from build123d import *

# Parameters (mm, degrees)
F1_DEPTH = 25.4


with BuildPart() as f1:
    # F0 (on Top) → F1 (new body)
    with BuildSketch(Plane.XY):
        with BuildLine():
            Line((24.443999, 9.764512), (32.35041, 21.669716))
            ThreePointArc((32.35041, 21.669716), (22.499546, 43.363489), (-1.08105, 39.955447))
            ThreePointArc((-1.08105, 39.955447), (-25.805681, 45.592397), (-38.979422, 23.923639))
            Line((-38.979422, 23.923639), (-25.198337, 5.393257))
            ThreePointArc((-25.198337, 5.393257), (-11.978415, 4.602569), (-0.762963, 11.645662))
            ThreePointArc((-0.762963, 11.645662), (11.502175, 6.171376), (24.443999, 9.764512))
        make_face()
        with BuildLine():
            ThreePointArc((24.443999, 9.764512), (29.506368, 14.980504), (32.35041, 21.669716))
            Line((32.35041, 21.669716), (24.443999, 9.764512))
        make_face()
        with BuildLine():
            Line((-25.198337, 5.393257), (-38.979422, 23.923639))
            ThreePointArc((-38.979422, 23.923639), (-34.759944, 12.671971), (-25.198337, 5.393257))
        make_face()
    extrude(amount=F1_DEPTH)


solid = f1.part
Part model, mm, in its own coordinate system. Coordinates: 2 decimals unless noted, no trailing zeros. Order: outer loops, then holes, each group sorted by start corner. A loop starts at its lowest first (then second) coordinate and runs counter-clockwise, first axis right, second up. Notation, with made-up numbers: (78.5, -27.5) - (109.5, -27.5) arc R35 cw to (109.5, 4.5) - close; hole circle Ø9 at (6, 67). An arc over 180 degrees is marked (long way). Use CSV: the item, a comma, the result in double quotes.
Item 1: Probe probe 1 along Y at (x, z) = (-18, 20.5); probe 2 along X at (y, z) = (44, 19); probe 3 along X at (y, z) = (37, 4.25). List the from-to ranges inside material, lowest first.
Solved:
probe 1,"y = 3.94 to 47.3"
probe 2,"x = -28.87 to -5.84, 4.73 to 21.23"
probe 3,"x = -35.82 to 29.46"
Item 2: Saw through at B-B on x = 26. Give the cut face in (y, z).
Solved:
outline,"(10.99, 0) - (40.93, 0) - (40.93, 25.4) - (10.99, 25.4) - close"
Item 3: Drop flat-ended pins along their axis: P1, Ø10, axis at y = 37.5, z = 9, coming from the -X side; P2, Ø6, axis at x = -6, z = 11, coming from the -Y side; P3, Ø1, axis at y = 32.5, z = 22, coming from the -X side. Give the stop position or say it passes through.
Solved:
P1,"stops at x = -37.92"
P2,"stops at y = 5.6"
P3,"stops at x = -38.08"
Item 4: Saw through at C-C on y = 15. Give the cut face in (x, z), and give its area (3 significant figures).
Solved:
outline,"(-36.27, 0) - (29.52, 0) - (29.52, 25.4) - (-36.27, 25.4) - close"
area,"1,670 mm²"
Item 5: Saw through at A-A on y = 8.5. Give the cut face in (x, z), and give its area (3 significant figures).
Solved:
outline,"(-30.68, 0) - (-4.03, 0) - (-4.03, 25.4) - (-30.68, 25.4) - close; (3.55, 0) - (22.41, 0) - (22.41, 25.4) - (3.55, 25.4) - close"
area,"1,160 mm²"
Item 6: Saw through at D-D on z = 8.75. Give the cut face in (x, y).
Solved:
outline,"(-38.98, 23.92) arc R21.69 ccw to (-25.2, 5.39) arc R21.69 ccw to (-0.76, 11.65) arc R19.84 ccw to (24.44, 9.76) arc R19.84 ccw to (32.35, 21.67) arc R19.84 ccw to (-1.08, 39.96) arc R21.69 ccw to start"
